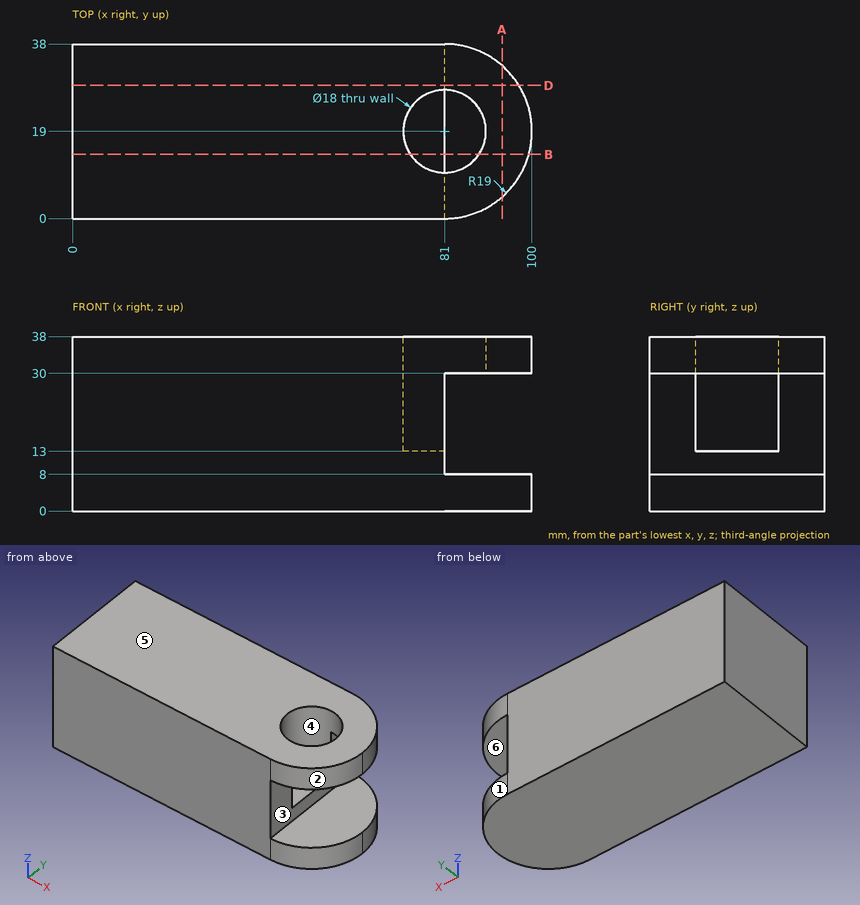
Part print with two shaded views. Sizes in mm from the minimum x, y, z corner. A direction names the side the tool comes from. Coordinates: 2 decimals unless noted, no trailing zeros. Write each loop counter-clockwise with the first axis right and the second up, starting at its lowest first coordinate (ties: lowest second). Pieces come first, ordered by that corner, then holes. Notation, with made-up numbers: (5, 46) -> (55, 46) arc R30 cw to (55, 70) -> close; hole circle Ø9 at (89.5, 54). An arc over 180 degrees is marked (long way). Return JSON: item names as keys, results as strings. Group by question number.
Q1. Which spindle directions (+Z, -Z, +X, -X, +Y, -Y) get a long thin tool onto all of the face, cutting with end or side? Do the marked faces 5 and 6. Say none if no direction does.
Q2. Cut at B-B, the plane y = 14. Give the cut face in (x, z).
Q3. Pull direction Y, two halves, no side cores. Call the marked faces 1, 2, 3 and 4: released by +Y, released by -Y, zero draft, split by the parting line, or undercut.
Q4. Cut at A-A, the plane x = 93.5. Give the cut face in (y, z).
Q5. Drill centre lines: line 1 (Y direction, x = 81, z = 30.25); line 2 (X direction, y = 2, z = 24); line 3 (Y direction, x = 83.5, z = 33). Where is each one in solid material? Low to high.
Q6. Flat gauge pins, fed straight in: pin 1 (6 mm diameter, centred on x = 28, y = 17, fed in from -Z); pin 2 (10 mm diameter, centred on y = 8.5, z = 30, fed in from +X); pin 3 (4.5 mm diameter, centred on x = 74.5, y = 19.5, fed in from +Z); pin 4 (1.5 mm diameter, centred on y = 5, z = 23, fed in from +X). Where does each tip first touch, or does it go through?
Q7. Cut at D-D, the plane y = 29. Give the cut face in (x, z).
Returned:
{
 "1": {"face 5": "+Z, +X, -X, +Y, -Y", "face 6": "+X, +Y, -Y"},
 "2": {"outline": "(0, 0) -> (99.33, 0) -> (99.33, 8) -> (81, 8) -> (81, 13) -> (73.52, 13) -> (73.52, 38) -> (0, 38) -> close; (88.48, 30) -> (99.33, 30) -> (99.33, 38) -> (88.48, 38) -> close"},
 "3": {"face 1": "released by +Y", "face 2": "released by -Y", "face 3": "zero draft", "face 4": "undercut"},
 "4": {"outline": "(4.69, 0) -> (33.31, 0) -> (33.31, 8) -> (4.69, 8) -> close; (4.69, 30) -> (33.31, 30) -> (33.31, 38) -> (4.69, 38) -> close"},
 "5": {"line 1": "y = 0 to 10, 28 to 38", "line 2": "x = 0 to 81", "line 3": "y = 0.17 to 10.35, 27.65 to 37.83"},
 "6": {"pin 1": "stops at z = 0", "pin 2": "stops at x = 99.19", "pin 3": "stops at z = 13", "pin 4": "stops at x = 81"},
 "7": {"outline": "(0, 0) -> (97.16, 0) -> (97.16, 8) -> (81, 8) -> (81, 30) -> (97.16, 30) -> (97.16, 38) -> (0, 38) -> close"}
}
